Input: part model. Units: mm. Frame: model coordinates. Give positions to 0.01 mm unless a question says otherwise; leave off trailing zeros. Write each loop counter-clockwise with the first axis right and the second up, starting at its lowest first coordinate (ties: lowest second). Pieces come first, ordered by that corner, then holes. Notation, with made-up numbers: (-21.5, 79.5) - (34.5, 79.5) arc R16 ccw to (34.5, 109.5) - close; hole circle Ø11 at (83, 76). An arc over 180 degrees is marked (long way). Answer as a JSON object with one key per item and string values. Group by question number.
from build123d import *

# Parameters (mm, degrees)
SKETCH_1_R      = 2
SKETCH_1_R_2    = 5
EXTRUDE_2_DEPTH = 2


with BuildPart() as part:
    # 草图1 → 凸台-拉伸2 (new body)
    with BuildSketch(Plane.XY):
        with BuildLine():
            Line((-37, -12.75), (-41, -12.75))
            Line((-41, -12.75), (-41, -9.5))
            Line((-41, -9.5), (-43, -9.5))
            Line((-43, -9.5), (-43, -4.5))
            Line((-43, -4.5), (-41, -4.5))
            Line((-41, -4.5), (-41, -1.5))
            Line((-41, -1.5), (-38.5, -1.5))
            Line((-38.5, -1.5), (-38.5, -3))
            Line((-38.5, -3), (-35.9, -3))
            Line((-35.9, -3), (-35.9, -1.5))
            Line((-35.9, -1.5), (-32.9, -1.5))
            Line((-32.9, -1.5), (-32.9, 1.5))
            Line((-32.9, 1.5), (-35.9, 1.5))
            Line((-35.9, 1.5), (-35.9, 3))
            Line((-35.9, 3), (-38.5, 3))
            Line((-38.5, 3), (-38.5, 1.5))
            Line((-38.5, 1.5), (-41, 1.5))
            Line((-41, 1.5), (-41, 4.5))
            Line((-41, 4.5), (-43, 4.5))
            Line((-43, 4.5), (-43, 9.5))
            Line((-43, 9.5), (-41, 9.5))
            Line((-41, 9.5), (-41, 12.75))
            Line((-41, 12.75), (-37, 12.75))
            Line((-37, 12.75), (-37, 14.75))
            Line((-37, 14.75), (-30, 14.75))
            Line((-30, 14.75), (-30, 12.75))
            Line((-30, 12.75), (-25.488968202, 12.75))
            Line((-25.488968202, 12.75), (-14.028482804, 5.790513304))
            ThreePointArc((-14.028482804, 5.790513304), (-11.304453577, 6.424059234), (-11.8771357, 9.161530853))
            Line((-11.8771357, 9.161530853), (-15.689334886, 16.190924706))
            ThreePointArc((-15.689334886, 16.190924706), (-15.886477166, 18.604361531), (-14.237063941, 20.37720625))
            ThreePointArc((-14.237063941, 20.37720625), (-0.042376251, 23.307851412), (14.159162664, 20.410588547))
            ThreePointArc((14.159162664, 20.410588547), (15.812739599, 18.641626787), (15.621272277, 16.227733118))
            Line((15.621272277, 16.227733118), (11.768369699, 9.083252425))
            ThreePointArc((11.768369699, 9.083252425), (11.351042044, 6.354326573), (14.057146467, 5.808251922))
            Line((14.057146467, 5.808251922), (25.488968202, 12.75))
            Line((25.488968202, 12.75), (30, 12.75))
            Line((30, 12.75), (30, 14.75))
            Line((30, 14.75), (37, 14.75))
            Line((37, 14.75), (37, 12.75))
            Line((37, 12.75), (41, 12.75))
            Line((41, 12.75), (41, 9.5))
            Line((41, 9.5), (43, 9.5))
            Line((43, 9.5), (43, 4.5))
            Line((43, 4.5), (41, 4.5))
            Line((41, 4.5), (41, 1.5))
            Line((41, 1.5), (38.5, 1.5))
            Line((38.5, 1.5), (38.5, 3))
            Line((38.5, 3), (35.9, 3))
            Line((35.9, 3), (35.9, 1.5))
            Line((35.9, 1.5), (32.9, 1.5))
            Line((32.9, 1.5), (32.9, -1.5))
            Line((32.9, -1.5), (35.9, -1.5))
            Line((35.9, -1.5), (35.9, -3))
            Line((35.9, -3), (38.5, -3))
            Line((38.5, -3), (38.5, -1.5))
            Line((38.5, -1.5), (41, -1.5))
            Line((41, -1.5), (41, -4.5))
            Line((41, -4.5), (43, -4.5))
            Line((43, -4.5), (43, -9.5))
            Line((43, -9.5), (41, -9.5))
            Line((41, -9.5), (41, -12.75))
            Line((41, -12.75), (37, -12.75))
            Line((37, -12.75), (37, -14.75))
            Line((37, -14.75), (30, -14.75))
            Line((30, -14.75), (30, -12.75))
            Line((30, -12.75), (25.488968202, -12.75))
            ThreePointArc((25.488968202, -12.75), (16.622058042, -19.246687746), (6.209460579, -22.769025255))
            ThreePointArc((6.209460579, -22.769025255), (3.920471276, -22.23446682), (2.719464237, -20.213871155))
            Line((2.719464237, -20.213871155), (2, -14.866068747))
            ThreePointArc((2, -14.866068747), (0, -12.997534789), (-2, -14.866068747))
            Line((-2, -14.866068747), (-2.719464237, -20.213871155))
            ThreePointArc((-2.719464237, -20.213871155), (-3.920471276, -22.23446682), (-6.209460579, -22.769025255))
            ThreePointArc((-6.209460579, -22.769025255), (-16.622058042, -19.246687746), (-25.488968202, -12.75))
            Line((-25.488968202, -12.75), (-30, -12.75))
            Line((-30, -12.75), (-30, -14.75))
            Line((-30, -14.75), (-37, -14.75))
            Line((-37, -14.75), (-37, -12.75))
        make_face()
        with Locations((0, 14.25)):
            Circle(SKETCH_1_R, mode=Mode.SUBTRACT)
        with Locations((12.340862004, -7.125)):
            Circle(SKETCH_1_R, mode=Mode.SUBTRACT)
        with Locations((-12.340862004, -7.125)):
            Circle(SKETCH_1_R, mode=Mode.SUBTRACT)
        Circle(SKETCH_1_R_2, mode=Mode.SUBTRACT)
    extrude(amount=EXTRUDE_2_DEPTH)


solid = part.part
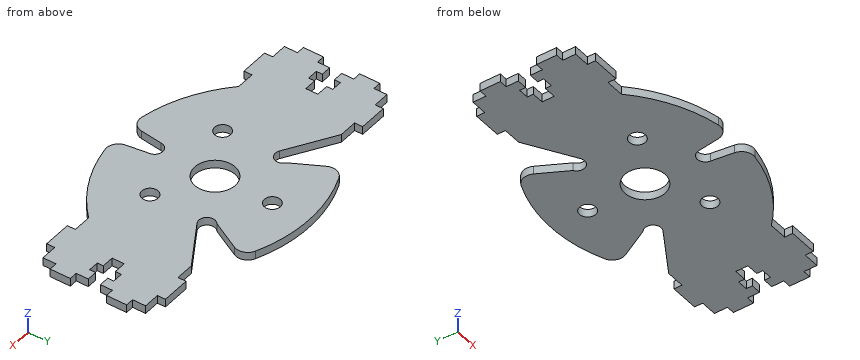
1) Cut plane D-D on z = 1.1. Count the separate pieces of the cut face and the enclosed holes in it, and give its area (3 significant figures).
2) Pin query (flat end, axial travel): P1, Ø0.6, axis at x = -39.5, z = 1, coming from the -Y side; P2, Ø1, axis at x = -12.5, z = 0.5, coming from the -Y side; P3, Ø1, axis at x = 34, z = 1, coming from the -Y side. Return the tip coordinate at first contact, or that it passes through.
3) Cut plane A-A on x = 0. Return the cut outline in (y, z), and give its area (3 significant figures).
4) Cut plane B-B on x = 35. Return the cut outline in (y, z).
5) Line query: line 1 along Y through (x, z) = (0, 0.5); line 2 along X through (y, z) = (8, 1.4); line 3 along X through (y, z) = (11.5, 0.8). Output: solid intervals per line, ascending. Write a range as from..to.
6) Cut plane C-C on y = 7.5. Return the cut outline in (x, z), and give its area (3 significant figures).
Filled in:
{
 "1": {"separate pieces": "1", "enclosed holes": "4", "area": "2,510 mm²"},
 "2": {"P1": "stops at y = -12.75", "P2": "stops at y = -21.25", "P3": "stops at y = -14.75"},
 "3": {"outline": "(-13, 0) - (-5, 0) - (-5, 2) - (-13, 2) - close; (5, 0) - (12.25, 0) - (12.25, 2) - (5, 2) - close; (16.25, 0) - (23.31, 0) - (23.31, 2) - (16.25, 2) - close", "area": "44.6 mm²"},
 "4": {"outline": "(-14.75, 0) - (-1.5, 0) - (-1.5, 2) - (-14.75, 2) - close; (1.5, 0) - (14.75, 0) - (14.75, 2) - (1.5, 2) - close"},
 "5": {"line 1": "y = -13..-5, 5..12.25, 16.25..23.31", "line 2": "x = -43..-17.67, -11.05..11.05, 17.67..43", "line 3": "x = -41..-23.43, -13.15..13.07, 23.43..41"},
 "6": {"outline": "(-43, 0) - (-16.84, 0) - (-16.84, 2) - (-43, 2) - close; (-10.99, 0) - (10.99, 0) - (10.99, 2) - (-10.99, 2) - close; (16.84, 0) - (43, 0) - (43, 2) - (16.84, 2) - close", "area": "149 mm²"}
}
